For this review, take the finished solid that the model builds, in its own axes (mm). Face numbers are marked on the shaded views. A direction names the side the tool comes from. Give positions to 0.01 mm unless a question says otherwise; leave off trailing zeros. Loops run counter-clockwise (first coordinate to the right, second up) from the corner with the lowest first, then second, coordinate; pieces in that order, holes last.
Autodesk Fusion 360 part; units mm, degrees
sketch "Sketch1" plane through (0, 0, 0) normal (0, 1, 0) x (1, 0, 0)
  line L0 (0, -85) -> (85, -85)
  line L1 (85, -85) -> (85, 85)
  line L2 (85, 85) -> (-85, 85)
  line L3 (-85, 85) -> (-85, -85)
  line L4 (-85, -85) -> (0, -85)
  dimension "d4" = 170
  dimension "d5" = 170
extrude "Extrude1" add sketch "Sketch1" along normal blind 20
sketch "Sketch2" plane through (0, 20, 0) normal (0, 1, 0) x (-1, 0, 0)
  line L0 (85, 85) -> (-85, 85)
  line L1 (-85, 85) -> (-85, -85)
  line L2 (-85, -85) -> (85, -85)
  line L3 (85, -85) -> (85, 85)
  line L4 (65, 0) -> (65, -20)
  line L5 (65, -20) -> (25, -20)
  line L6 (25, -20) -> (25, 20)
  line L7 (25, 20) -> (65, 20)
  line L8 (65, 20) -> (65, 0)
  line L9 (-25, 0) -> (-25, -20)
  line L10 (-25, -20) -> (-65, -20)
  line L11 (-65, -20) -> (-65, 20)
  line L12 (-65, 20) -> (-25, 20)
  line L13 (-25, 20) -> (-25, 0)
  dimension "d13" = 40
  dimension "d14" = 40
  dimension "d17" = 40
  dimension "d18" = 40
extrude "Extrude2" add sketch "Sketch2" along normal blind 10 contours L4 L5 L6 L7 L8 | L9 L10 L11 L12 L13
sketch "Sketch3" plane through (0, 30, 0) normal (0, 1, 0) x (-1, 0, 0)
  line L0 (-25, 20) -> (-65, 20)
  line L1 (-65, 20) -> (-65, -20)
  line L2 (-65, -20) -> (-25, -20)
  line L3 (-25, -20) -> (-25, 20)
  line L4 (-28, 0) -> (-28, -17)
  line L5 (-28, -17) -> (-62, -17)
  line L6 (-62, -17) -> (-62, 17)
  line L7 (-62, 17) -> (-28, 17)
  line L8 (-28, 17) -> (-28, 0)
  dimension "d24" = 34
  dimension "d25" = 34
extrude "Extrude3" cut sketch "Sketch3" against normal blind 50 contours L4 L5 L6 L7 L8
sketch "Sketch4" plane through (0, 30, 0) normal (0, 1, 0) x (-1, 0, 0)
  line L0 (65, 20) -> (25, 20)
  line L1 (25, 20) -> (25, -20)
  line L2 (25, -20) -> (65, -20)
  line L3 (65, -20) -> (65, 20)
  line L4 (62, 0) -> (62, -17)
  line L5 (62, -17) -> (28, -17)
  line L6 (28, -17) -> (28, 17)
  line L7 (28, 17) -> (62, 17)
  line L8 (62, 17) -> (62, 0)
  dimension "d31" = 34
  dimension "d32" = 34
extrude "Extrude4" cut sketch "Sketch4" against normal blind 50 contours L4 L5 L6 L7 L8
fillet "Fillet1" radius 3 1 edges at (-45, 20, 20)
fillet "Fillet2" radius 3 1 edges at (-25, 20, 1.5)
fillet "Fillet3" radius 3 1 edges at (45, 20, 20)
fillet "Fillet4" radius 3 1 edges at (65, 20, 1.5)
fillet "Fillet5" radius 3 4 edges at (25, 20, 1.5) (46.5, 20, -20) (-43.5, 20, -20) (-65, 20, 1.5)
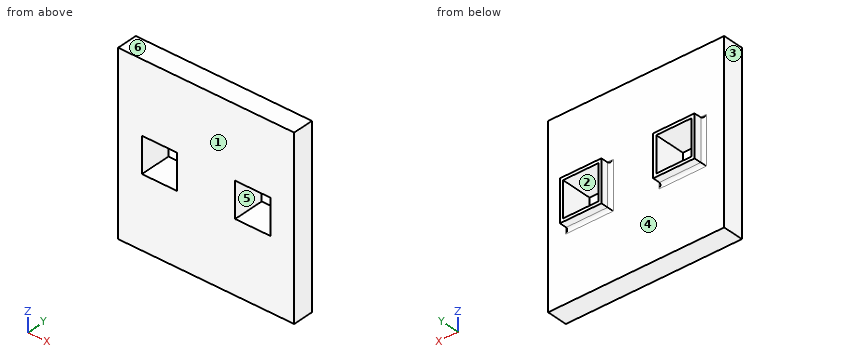
Q1. Consider section A-A on x = 33.5. Give the boundary of the cut face in (y, z).
Answers:
outline: (0, -85) - (20, -85) - (20, -23) arc R3 cw to (23, -20) - (30, -20) - (30, -17) - (0, -17) - close; (0, 17) - (30, 17) - (30, 20) - (23, 20) arc R3 cw to (20, 23) - (20, 85) - (0, 85) - close
Q2. For pin 1 Ø3.5 at (x, y) = (50.5, 28) entering from -Z; pin 2 Ø1.5 at (x, z) = (67, 7) entering from +Y; pin 3 Ø2 at (x, y) = (38, 27) entering from +Z, all flat-tipped, find the tip position at first contact; note any pin that passes through.
Answers:
pin 1: stops at z = -20
pin 2: stops at y = 20.56
pin 3: stops at z = 20
Q3. Consider section B-B on y = 8. Give the boundary of the cut face in (x, z), plus the area to 3 significant figures.
Answers:
outline: (-85, -85) - (85, -85) - (85, 85) - (-85, 85) - close; hole (-62, -17) - (-28, -17) - (-28, 17) - (-62, 17) - close; hole (28, -17) - (62, -17) - (62, 17) - (28, 17) - close
area: 26,600 mm2
Q4. For probe 1 along X at (y, z) = (17.5, -14.5); probe 2 along Z at (x, y) = (-36, 14); probe 3 along Y at (x, z) = (53, 61), list the stretches that pass through material, from the lowest coordinate up.
Answers:
probe 1: x = -85 to -62, -28 to 28, 62 to 85
probe 2: z = -85 to -17, 17 to 85
probe 3: y = 0 to 20
Q5. Consider section D-D on x = 72.5. Give the boundary of the cut face in (y, z).
Answers:
outline: (0, -85) - (20, -85) - (20, 85) - (0, 85) - close
Q6. Mouldability with a two-part tool opening along X and no side actions: class the marked faces 1, 2 and 3 as +X half, -X half, draft (parallel to the pull), parting line (faces both ways), or undercut.
Answers:
face 1: draft
face 2: undercut
face 3: -X half
Q7. Machinability: for the marked faces 4, 5 and 6, which of the approach directions +Z, -Z, +X, -X, +Y, -Y give a long, thin tool a straight path to every point of the face, cutting with its end or side? Answer none if there is none.
Answers:
face 4: +Y
face 5: +Y, -Y
face 6: +Z, +X, -X, +Y, -Y
Q8. Consider section C-C on z = 13. Give the boundary of the cut face in (x, y).
Answers:
outline: (-85, 0) - (-62, 0) - (-62, 30) - (-65, 30) - (-65, 23) arc R3 cw to (-68, 20) - (-85, 20) - close; (-28, 0) - (28, 0) - (28, 30) - (25, 30) - (25, 23) arc R3 cw to (22, 20) - (-22, 20) arc R3 cw to (-25, 23) - (-25, 30) - (-28, 30) - close; (62, 0) - (85, 0) - (85, 20) - (68, 20) arc R3 cw to (65, 23) - (65, 30) - (62, 30) - close
